```python
from build123d import *

# Parameters (mm, degrees)
SKETCH1_R           = 2
SKETCH1_R_2         = 2.38125
SKETCH1_R_3         = 1.97
BASE_DEPTH          = 6
ALL_CUTS_DEPTH      = 76.612498967
ALL_CUTS_DEPTH_BACK = 76.612498967
SKETCH2_W           = 5
SKETCH2_H           = 40
SKETCH2_W_2         = 6
SKETCH2_H_2         = 20
SKETCH2_H_3         = 30
SKETCH2_W_3         = 8
SKETCH3_W           = 16
SKETCH3_H           = 24
SKETCH3_W_2         = 8
SKETCH3_H_2         = 20
BOSS_EXTRUDE1_DEPTH = 15
SKETCH4_R           = 2.38125
CUT_EXTRUDE1_DEPTH  = 78.053552806
FILLET1_R           = 2.5
FILLET2_R           = 8
FILLET3_R           = 8
BOSS_EXTRUDE2_DEPTH = 1


with BuildPart() as part:
    # Sketch1 → BASE (new, symmetric)
    with BuildSketch(Plane(origin=(0, 0, 0), x_dir=(0, 0, -1), z_dir=(1, 0, 0))):
        with BuildLine():
            Line((-67.5, 7.5), (67.5, 7.5))
            ThreePointArc((67.5, 7.5), (75, 0), (67.5, -7.5))
            Line((67.5, -7.5), (-67.5, -7.5))
            ThreePointArc((-67.5, -7.5), (-75, 0), (-67.5, 7.5))
        make_face()
        with Locations((-67.5, 0)):
            Circle(SKETCH1_R, mode=Mode.SUBTRACT)
        Circle(SKETCH1_R_2, mode=Mode.SUBTRACT)
        with Locations((67.5, 0)):
            Circle(SKETCH1_R_3, mode=Mode.SUBTRACT)
    extrude(amount=BASE_DEPTH, both=True)

    # Sketch2 → All_Cuts (cut, two sides: drawn at the far end of the back side and taken through both)
    with BuildSketch(Plane(origin=(0, 0, 0), x_dir=(1, 0, 0), z_dir=(0, 1, 0)).offset(-ALL_CUTS_DEPTH_BACK)):
        with Locations((0, -75)):
            Rectangle(SKETCH2_W, SKETCH2_H)
        with Locations((-6, -30)):
            Rectangle(SKETCH2_W_2, SKETCH2_H_2)
        with Locations((6, -30)):
            Rectangle(SKETCH2_W_2, SKETCH2_H_2)
        with Locations((6, 60)):
            Rectangle(SKETCH2_W_2, SKETCH2_H_3)
        with Locations((-6, 60)):
            Rectangle(SKETCH2_W_2, SKETCH2_H_3)
        Rectangle(SKETCH2_W_3, SKETCH2_H_2)
    extrude(amount=ALL_CUTS_DEPTH + ALL_CUTS_DEPTH_BACK, mode=Mode.SUBTRACT)

    # Sketch3 → Boss-Extrude1 (add, through all)
    with BuildSketch(Plane.XZ.offset(7.5)):
        Rectangle(SKETCH3_W, SKETCH3_H)
        Rectangle(SKETCH3_W_2, SKETCH3_H_2, mode=Mode.SUBTRACT)
    extrude(amount=-BOSS_EXTRUDE1_DEPTH)

    # Sketch4 → Cut-Extrude1 (cut, through all)
    with BuildSketch(Plane.ZY.offset(8)):
        Circle(SKETCH4_R)
    extrude(amount=-CUT_EXTRUDE1_DEPTH, mode=Mode.SUBTRACT)

    # Fillet1
    fillet1_edges = [part.edges().sort_by_distance(p)[0] for p in [
        (3, 0, 20),
        (3, 0, 40),
        (-3, 0, 40),
        (-3, 0, 20),
        (3, 0, -45),
        (-3, 0, -45),
    ]]
    fillet(fillet1_edges, radius=FILLET1_R)

    # Fillet2
    # the kernel refuses this fillet: 8 mm, written as the material it adds along each edge
    with BuildSketch(Plane(origin=(-6, -7.5, -12), x_dir=(0, 0, -1), z_dir=(0, 1, 0))) as fillet2_piece_1:
        with BuildLine():
            CenterArc((5.291502622, 8), FILLET2_R, 228.590377891, 41.409622109)
            Line((0, 2), (-0.105830052, 1.88))
            ThreePointArc((-0.105830052, 1.88), (-0.16, 1), (-0.16, 0))
            Line((-0.16, 0), (0, -0.16))
            Line((0, -0.16), (5.291502622, -0.16))
            Line((5.291502622, -0.16), (5.291502622, 0))
        make_face()
    extrude(amount=15)
    with BuildSketch(Plane(origin=(6, -7.5, -12), x_dir=(1, 0, 0), z_dir=(0, 1, 0))) as fillet2_piece_2:
        with BuildLine():
            CenterArc((8, 5.291502622), FILLET2_R, 180, 41.409622109)
            Line((0, 5.291502622), (-0.16, 5.291502622))
            Line((-0.16, 5.291502622), (-0.16, 0))
            Line((-0.16, 0), (0, -0.16))
            ThreePointArc((0, -0.16), (1, -0.16), (1.88, -0.105830052))
            Line((1.88, -0.105830052), (2, 0))
        make_face()
    extrude(amount=15)
    with BuildSketch(Plane(origin=(6, 7.5, 12), x_dir=(0, 0, 1), z_dir=(0, -1, 0))) as fillet2_piece_3:
        with BuildLine():
            CenterArc((5.291502622, -8), FILLET2_R, 90, 41.409622109)
            Line((0, -2), (-0.105830052, -1.88))
            ThreePointArc((-0.105830052, -1.88), (-0.16, -1), (-0.16, 0))
            Line((-0.16, 0), (0, 0.16))
            Line((0, 0.16), (5.291502622, 0.16))
            Line((5.291502622, 0.16), (5.291502622, 0))
        make_face()
    extrude(amount=15)
    with BuildSketch(Plane(origin=(-6, 7.5, 12), x_dir=(-1, 0, 0), z_dir=(0, -1, 0))) as fillet2_piece_4:
        with BuildLine():
            CenterArc((8, -5.291502622), FILLET2_R, 138.590377891, 41.409622109)
            Line((0, -5.291502622), (-0.16, -5.291502622))
            Line((-0.16, -5.291502622), (-0.16, 0))
            Line((-0.16, 0), (0, 0.16))
            ThreePointArc((0, 0.16), (1, 0.16), (1.88, 0.105830052))
            Line((1.88, 0.105830052), (2, 0))
        make_face()
    extrude(amount=15)

    # Fillet3
    fillet3_edges = [part.edges().sort_by_distance(p)[0] for p in [
        (8, 0, -12),
        (-8, 0, -12),
        (-6, 0, 20),
        (6, 0, 20),
        (-6, 0, -45),
        (6, 0, -45),
        (6, 0, 40),
        (-6, 0, 40),
    ]]
    fillet(fillet3_edges, radius=FILLET3_R)

    # Sketch5 → Boss-Extrude2 (add)
    # profile 1 of 2: a face of its own
    with BuildSketch(Plane(origin=(0, 7.5, 0), x_dir=(1, 0, 0), z_dir=(0, 1, 0))):
        Polygon((-3.52782764, 31.96394622), (-2.549420522, 31.96394622), (-2.549420522, 26.672279553), (-3.024313685, 26.672279553), (-3.024313685, 31.421211177), (-3.838416249, 31.421211177), align=None)
    # profile 2 of 2: a face of its own
    with BuildSketch(Plane(origin=(0, 7.5, 0), x_dir=(1, 0, 0), z_dir=(0, 1, 0))):
        with BuildLine():
            Line((1.8603017, 32.09962998), (2.226011836, 31.812362018))
            Line((2.226011836, 31.812362018), (0.827833083, 29.674282758))
            add(Edge.make_bspline(
                [(0.827833083, 29.674282758), (0.920921478, 29.689120381), (1.102500918, 29.718062841), (1.286296979, 29.722837354), (1.375868273, 29.725164168)],
                knots=[0, 0, 0, 0, 1.025318673, 2, 2, 2, 2], degree=3))
            add(Edge.make_bspline(
                [(1.375868273, 29.725164168), (1.4296505, 29.723718619), (1.535519212, 29.720873097), (1.690953306, 29.698974894), (1.840312769, 29.664465498), (1.98297854, 29.614161016), (2.119462691, 29.549901504), (2.250548456, 29.472886784), (2.373771734, 29.3791401), (2.49071935, 29.274418084), (2.596896033, 29.15842931), (2.690900307, 29.035358241), (2.769862242, 28.9053331), (2.833927576, 28.768419743), (2.883676619, 28.624829219), (2.919943654, 28.474745247), (2.941381848, 28.318064331), (2.944293006, 28.211508043), (2.945771785, 28.157380715)],
                knots=[0, 0, 0, 0, 1.04369286, 2.054478336, 3.041073146, 4.015093852, 4.984733326, 5.965804835, 6.960378782, 7.985147595, 9.009457201, 10.008161701, 10.986880575, 11.956520048, 12.937015923, 13.931873656, 14.949455224, 16, 16, 16, 16], degree=3))
            add(Edge.make_bspline(
                [(2.945771785, 28.157380715), (2.943620186, 28.083328067), (2.939386349, 27.937609982), (2.897198467, 27.725373771), (2.831642813, 27.523182944), (2.737938693, 27.334265649), (2.621548661, 27.158880812), (2.479614682, 27.003478977), (2.31717036, 26.864882611), (2.133493892, 26.748985104), (1.935822982, 26.654335253), (1.728159843, 26.586352089), (1.512521181, 26.54449732), (1.366161833, 26.539250099), (1.292125952, 26.536595792)],
                knots=[0, 0, 0, 0, 1.031375318, 2.029502543, 3.004789286, 3.987476834, 4.960371455, 5.9300674, 6.912260825, 7.929083631, 8.949397511, 9.960523116, 10.96833055, 12, 12, 12, 12], degree=3))
            add(Edge.make_bspline(
                [(1.292125952, 26.536595792), (1.220920226, 26.538906294), (1.07987415, 26.543482993), (0.872391235, 26.584252923), (0.673026911, 26.6503339), (0.483177966, 26.741372154), (0.307312278, 26.856364429), (0.149974946, 26.994797875), (0.011950478, 27.153713376), (-0.102915914, 27.333086282), (-0.194021377, 27.525838956), (-0.26234424, 27.726827276), (-0.302252846, 27.935318915), (-0.307829593, 28.076653494), (-0.310638471, 28.14784045)],
                knots=[0, 0, 0, 0, 1.012016664, 2.004627821, 2.994792927, 3.992885782, 4.990978636, 5.973936114, 6.964471063, 7.975201453, 8.993600317, 9.990122807, 10.98767138, 12, 12, 12, 12], degree=3))
            add(Edge.make_bspline(
                [(-0.310638471, 28.14784045), (-0.308852239, 28.202336427), (-0.305205094, 28.3136068), (-0.279739491, 28.482129795), (-0.238820099, 28.654564168), (-0.192993894, 28.800847294), (-0.144574221, 28.920683167), (-0.10427812, 29.017299159), (-0.054122197, 29.116723638), (-0.000641014, 29.222365921), (0.060979491, 29.331503421), (0.127980532, 29.445960159), (0.202214528, 29.563915835), (0.254254536, 29.643962416), (0.280857923, 29.684883052)],
                knots=[0, 0, 0, 0, 1.173818275, 2.396712641, 3.66331629, 4.989737886, 5.693666774, 6.447286557, 7.243889047, 8.091586357, 8.998013824, 9.943181721, 10.948533338, 12, 12, 12, 12], degree=3))
            Line((0.280857923, 29.684883052), (1.8603017, 32.09962998))
        make_face()
        with BuildLine():
            add(Edge.make_bspline(
                [(1.276225511, 29.182429126), (1.235914736, 29.181252798), (1.157176083, 29.178955087), (1.041655349, 29.165612147), (0.9323246, 29.140485703), (0.827735362, 29.108484225), (0.729843001, 29.06448317), (0.637936065, 29.011034617), (0.551659141, 28.948107359), (0.471915914, 28.876592887), (0.399617138, 28.798294313), (0.33735519, 28.714429678), (0.283648704, 28.627020109), (0.239982145, 28.535335268), (0.205979292, 28.439410203), (0.181383246, 28.3396861), (0.167694836, 28.235494232), (0.165417558, 28.164839139), (0.164254691, 28.128759922)],
                knots=[0, 0, 0, 0, 1.129588631, 2.206414736, 3.251139165, 4.268635594, 5.265702196, 6.250456724, 7.242448911, 8.251968645, 9.246821453, 10.222880186, 11.173611482, 12.116736599, 13.062300278, 14.020270554, 14.989073742, 16, 16, 16, 16], degree=3))
            add(Edge.make_bspline(
                [(0.164254691, 28.128759922), (0.16520169, 28.093003404), (0.167058614, 28.022890197), (0.18391986, 27.919567866), (0.209675282, 27.820137588), (0.247987547, 27.725111957), (0.293687723, 27.633042523), (0.354020773, 27.547264175), (0.420872342, 27.462567164), (0.500782455, 27.385457797), (0.586542778, 27.313707901), (0.678166025, 27.250993708), (0.773657869, 27.197341993), (0.874307519, 27.155294262), (0.97868698, 27.120786114), (1.087665913, 27.096502688), (1.201320111, 27.082773797), (1.278309232, 27.080493552), (1.317566657, 27.079330835)],
                knots=[0, 0, 0, 0, 0.989467248, 1.94019797, 2.891935182, 3.827694429, 4.772920941, 5.730924762, 6.725747692, 7.756678648, 8.79901574, 9.819492441, 10.826891316, 11.826466727, 12.835195252, 13.867842842, 14.912794438, 16, 16, 16, 16], degree=3))
            add(Edge.make_bspline(
                [(1.317566657, 27.079330835), (1.356824018, 27.080493643), (1.433813013, 27.082774067), (1.547468125, 27.096501662), (1.656443678, 27.120789879), (1.760835423, 27.155280615), (1.86143973, 27.19739262), (1.956848059, 27.250659927), (2.047604819, 27.314093582), (2.13342144, 27.385335181), (2.212998942, 27.463006041), (2.281453876, 27.546508121), (2.33993924, 27.633735796), (2.387464737, 27.724749273), (2.425355023, 27.820195046), (2.451241051, 27.919552474), (2.468067476, 28.022894227), (2.469929184, 28.093004765), (2.470878623, 28.128759922)],
                knots=[0, 0, 0, 0, 1.087397944, 2.132534446, 3.165364764, 4.174271784, 5.174024072, 6.181601208, 7.194203697, 8.236725232, 9.267838612, 10.269026844, 11.221737037, 12.171628256, 13.107553087, 14.05945871, 15.010357665, 16, 16, 16, 16], degree=3))
            add(Edge.make_bspline(
                [(2.470878623, 28.128759922), (2.470046632, 28.164886207), (2.468413705, 28.235790356), (2.449944355, 28.339639493), (2.424329099, 28.439916888), (2.385649993, 28.535992311), (2.335399503, 28.62748663), (2.274192447, 28.714862026), (2.203386061, 28.798788385), (2.121595733, 28.87674644), (2.032559308, 28.948028332), (1.937890506, 29.010953137), (1.838848689, 29.064058757), (1.735534276, 29.108368304), (1.626763489, 29.140344295), (1.514292381, 29.165522413), (1.396682455, 29.178920939), (1.316889249, 29.181244836), (1.276225511, 29.182429126)],
                knots=[0, 0, 0, 0, 0.978206639, 1.919901502, 2.851605144, 3.780102724, 4.718870031, 5.675451981, 6.667674623, 7.690630536, 8.733308323, 9.756129687, 10.767539656, 11.776269907, 12.797430371, 13.836405707, 14.897401972, 16, 16, 16, 16], degree=3))
        make_face(mode=Mode.SUBTRACT)
    extrude(amount=BOSS_EXTRUDE2_DEPTH)


solid = part.part
```
Model file for the job. Use its own axes, mm. A direction names the side the tool comes from. Coordinates: 2 decimals unless noted, no trailing zeros. Write each loop counter-clockwise with the first axis right and the second up, starting at its lowest first coordinate (ties: lowest second). Pieces come first, ordered by that corner, then holes. Notation, with made-up numbers: (-30, 13.5) - (-13, 13.5) arc R15 cw to (-13, 35.5) - close; hole circle Ø3 at (33.5, 75). An arc over 180 degrees is marked (long way). One line per question, with ' | ' between items. Start each with the question number.
Q1. Cut at B-B, the plane y = 0. Give the number of separate pieces and of enclosed holes in the cut face, then the cut area to 3 significant figures.
Q2. Pull direction Z, two halves, no side cores. Call faces 4 (the face through (-4.274, 0.601, 65.592)), 5 (the face through (6.727, 0.105, 13.959)), 6 (the face through (0, 0, -10)), 7 (the face through (0, 0, -75)): pulls with the +Z half, pulls with the -Z half, needs draft (parallel to the pull), parting line crosses it, or undercut.
Q3. Cut at C-C, the plane z = -23. List the corners of the cut face in (x, y), then the cut area to 3 significant figures.
Q4. Drill centre lines: line 1 (Z direction, x = -1.45, y = 0); line 2 (Y direction, x = -4.4, z = 67.5); line 3 (X direction, y = 4, z = -7). Where is each one in solid material? Low to high. Write a range as [from, to].
Q5. Cut at A-A, the plane z = 0. List the corners of the cut face in (x, y).
Q6. 3-axis set-ups, long thin cutter, end or side, ignore diameter. For faces 1 (the face through (6, 0, -29)), 2 (the face through (-3, 0, -61)), 3 (the face through (-4, -2, 2)): which of +Z, -Z, +X, -X, +Y, -Y reach the whole face in a straight line?
Q7. Pin check, flat tips, straight feed: pin 1 (2 mm diameter, centred on y = -5.5, z = 55.5, fed in from -X); pin 2 (8 mm diameter, centred on x = -3.5, y = 6.5, fed in from -Z); pin 3 (5 mm diameter, centred on y = 3.5, z = -18, fed in from +X); pin 4 (5.5 mm diameter, centred on x = 0.5, y = 1.5, fed in from +Z). Stop position of each tip, or through.
Answer below:
1) separate pieces: 5 | enclosed holes: 0 | area: 1,250 mm^2
2) face 4: undercut | face 5: pulls with the +Z half | face 6: undercut | face 7: pulls with the -Z half
3) outline: (-6, -7.5) - (6, -7.5) - (6, 7.5) - (-6, 7.5) - close | area: 180 mm^2
4) line 1: [-75, -69.47], [-65.53, -10], [10, 55] | line 2: [-7.5, -2], [2, 7.5] | line 3: [-8, -4], [4, 8]
5) outline: (-8, -7.5) - (-4, -7.5) - (-4, -2.38) - (-8, -2.38) - close; (-8, 2.38) - (-4, 2.38) - (-4, 7.5) - (-8, 7.5) - close; (4, -7.5) - (8, -7.5) - (8, -2.38) - (4, -2.38) - close; (4, 2.38) - (8, 2.38) - (8, 7.5) - (4, 7.5) - close
6) face 1: -Z, +X, +Y, -Y | face 2: -Z, -X, +Y, -Y | face 3: +Y, -Y
7) pin 1: x = -6 | pin 2: z = -74.56 | pin 3: x = 6.2 | pin 4: z = 75
